```python
from build123d import *

# Parameters (mm, degrees)
SKETCH_W   = 175
SKETCH_H   = 170
SKETCH_R   = 3
SKETCH_R_2 = 1.025
SKETCH_W_2 = 145
SKETCH_H_2 = 80
SKETCH_W_3 = 144.774735
SKETCH_H_3 = 61.033017
PAD_DEPTH  = 3.5


with BuildPart() as part:
    # Sketch → Pad (new body)
    with BuildSketch(Plane.XY):
        with Locations((81.49518, -75)):
            Rectangle(SKETCH_W, SKETCH_H)
        Circle(SKETCH_R, mode=Mode.SUBTRACT)
        with Locations((0, -154.94)):
            Circle(SKETCH_R, mode=Mode.SUBTRACT)
        with Locations((157.48, -22.86)):
            Circle(SKETCH_R, mode=Mode.SUBTRACT)
        with Locations((157.48, -154.94)):
            Circle(SKETCH_R, mode=Mode.SUBTRACT)
        with Locations((22, 2)):
            Circle(SKETCH_R_2, mode=Mode.SUBTRACT)
        with Locations((156, 2)):
            Circle(SKETCH_R_2, mode=Mode.SUBTRACT)
        with Locations((22, -67)):
            Circle(SKETCH_R_2, mode=Mode.SUBTRACT)
        with Locations((156, -67)):
            Circle(SKETCH_R_2, mode=Mode.SUBTRACT)
        with Locations((78.558894, -111.02028)):
            Rectangle(SKETCH_W_2, SKETCH_H_2, mode=Mode.SUBTRACT)
        with Locations((78.48973, -32.597599)):
            Rectangle(SKETCH_W_3, SKETCH_H_3, mode=Mode.SUBTRACT)
    extrude(amount=PAD_DEPTH)


solid = part.part
```
Verification items for the finished model (mm, model axes). Coordinates: 2 decimals unless noted, no trailing zeros. Order: outer loops, then holes, each group sorted by start corner. A loop starts at its lowest first (then second) coordinate and runs counter-clockwise, first axis right, second up. Notation, with made-up numbers: (48, -30) -> (75, -30) arc R12 cw to (75, -20) -> close; hole circle Ø8 at (34.5, -38.75). An arc over 180 degrees is marked (long way). Put each result on its own line as item: value. Start each with the question number.
1) Cross-section at B-B (z = 1.3). State how many separate pieces and enclosed holes the cut face has, plus the area to 3 significant figures.
2) Cross-section at D-D (x = 35.5). Enter the section's corners in (y, z).
3) Cross-section at A-A (x = 0). Enter the section's corners in (y, z), plus the area to 3 significant figures.
4) Release check for a two-part mould opening along Y. For faces 1 (the flat face through (88, -68, 0)), 2 (the cylindrical face through (-3, 0, 2)) record: pulls with the +Y half, pulls with the -Y half, needs draft (parallel to the pull), parting line crosses it, or undercut.
5) Material ranges on L1, parallel to Y at x = 109, z = 2.55; L2, parallel to Y at x = 157.48, z = 1.45; L3, parallel to X at y = -154.94, z = 0.7, recorded low to high.
6) Cross-section at C-C (y = -13.5). Enter the section's corners in (x, z), plus the area to 3 significant figures.
Geometry check:
1. separate pieces: 1
1. enclosed holes: 10
1. area: 9,190 mm^2
2. outline: (-160, 0) -> (-151.02, 0) -> (-151.02, 3.5) -> (-160, 3.5) -> close; (-71.02, 0) -> (-63.11, 0) -> (-63.11, 3.5) -> (-71.02, 3.5) -> close; (-2.08, 0) -> (10, 0) -> (10, 3.5) -> (-2.08, 3.5) -> close
3. outline: (-160, 0) -> (-157.94, 0) -> (-157.94, 3.5) -> (-160, 3.5) -> close; (-151.94, 0) -> (-3, 0) -> (-3, 3.5) -> (-151.94, 3.5) -> close; (3, 0) -> (10, 0) -> (10, 3.5) -> (3, 3.5) -> close
3. area: 553 mm^2
4. face 1: needs draft
4. face 2: undercut
5. L1: y = -160 to -151.02, -71.02 to -63.11, -2.08 to 10
5. L2: y = -160 to -157.94, -151.94 to -25.86, -19.86 to 10
5. L3: x = -6 to -3, 3 to 154.48, 160.48 to 169
6. outline: (-6, 0) -> (6.1, 0) -> (6.1, 3.5) -> (-6, 3.5) -> close; (150.88, 0) -> (169, 0) -> (169, 3.5) -> (150.88, 3.5) -> close
6. area: 106 mm^2
